Part model, mm, in its own coordinate system. Round coordinates to 2 decimals unless told otherwise and drop trailing zeros. Order: outer loops, then holes, each group sorted by start corner. A loop starts at its lowest first (then second) coordinate and runs counter-clockwise, first axis right, second up. Notation, with made-up numbers: M 71.5,-21 L 101.5,-21 A20 cw 101.5,2 Z; hole C 79,-31 d6. An arc over 180 degrees is marked long. Write each question's results on one line, items separated by ' | '. Start each with the question number.
1. Probe L1, parallel to Z at x = 24, y = 3.75; L2, parallel to X at y = 3, z = 48; L3, parallel to Z at x = 40, y = 6.5. List the from-to ranges inside material, lowest first. Write a range as [from, to].
2. Band-saw the part on D-D, the plane z = -54. List the corners of the cut face in (x, y), then the cut area to 3 significant figures.
3. Band-saw the part on A-A, the plane x = 76. List the corners of the cut face in (y, z).
4. Band-saw the part on B-B, the plane y = 4.5. List the corners of the cut face in (x, z).
5. Band-saw the part on C-C, the plane z = 19. List the corners of the cut face in (x, y).
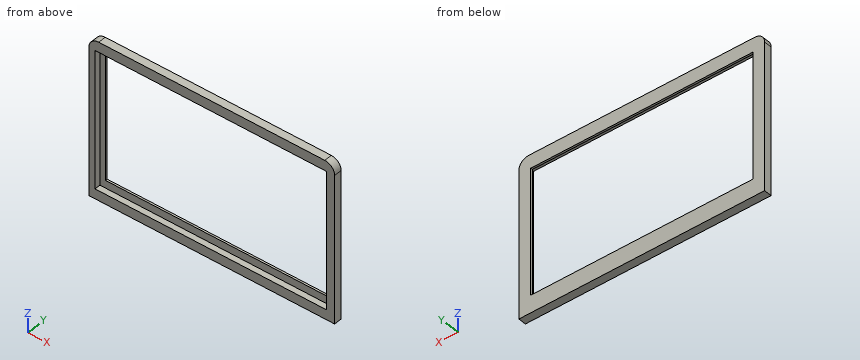
```python
from build123d import *

# Parameters (mm, degrees)
SKETCH_1_W          = 250
SKETCH_1_H          = 156
SKETCH_1_W_2        = 226
SKETCH_1_H_2        = 128
EXTRUDE_1_DEPTH     = 8
SKETCH_2_W          = 235.5
SKETCH_2_H          = 139.5
CUT_EXTRUDE_3_DEPTH = 6
SKETCH_11_W         = 250
SKETCH_11_H         = 8
EXTRUDE_3_DEPTH     = 3.75
CUT_EXTRUDE_4_DEPTH = 10


with BuildPart() as part:
    # 草图1 → 凸台-拉伸1 (new body)
    with BuildSketch(Plane(origin=(0, 0, 0), x_dir=(1, 0, 0), z_dir=(0, 1, 0))):
        with Locations((25.659327926, -14.898030127)):
            Rectangle(SKETCH_1_W, SKETCH_1_H)
        with Locations((25.659327926, -14.898030127)):
            Rectangle(SKETCH_1_W_2, SKETCH_1_H_2, mode=Mode.SUBTRACT)
    extrude(amount=EXTRUDE_1_DEPTH)

    # 草图2 → 切除-拉伸3 (cut)
    with BuildSketch(Plane.XZ):
        with Locations((24.659327926, 12.898030127)):
            Rectangle(SKETCH_2_W, SKETCH_2_H)
    extrude(amount=-CUT_EXTRUDE_3_DEPTH, mode=Mode.SUBTRACT)

    # 草图11 → 凸台-拉伸3 (add)
    with BuildSketch(Plane(origin=(0, 0, -63.101969873), x_dir=(-1, 0, 0), z_dir=(0, 0, -1))):
        with Locations((-25.659327926, 4)):
            Rectangle(SKETCH_11_W, SKETCH_11_H)
    extrude(amount=EXTRUDE_3_DEPTH)

    # 草图12 → 切除-拉伸4 (cut)
    with BuildSketch(Plane(origin=(0, 8, 0), x_dir=(1, 0, 0), z_dir=(0, 1, 0))):
        with BuildLine():
            Line((-99.340672074, -82.898030127), (-99.340672074, -92.898030127))
            Line((-99.340672074, -92.898030127), (-89.340672074, -92.898030127))
            ThreePointArc((-89.340672074, -92.898030127), (-96.411739886, -89.969097939), (-99.340672074, -82.898030127))
        make_face()
        with BuildLine():
            Line((150.659327926, -82.898030127), (150.659327926, -92.898030127))
            Line((150.659327926, -92.898030127), (140.659327926, -92.898030127))
            ThreePointArc((140.659327926, -92.898030127), (147.730395738, -89.969097939), (150.659327926, -82.898030127))
        make_face()
    extrude(amount=-CUT_EXTRUDE_4_DEPTH, mode=Mode.SUBTRACT)


solid = part.part
```
Solution:
1) L1: [-66.85, -56.85], [82.65, 92.9] | L2: [-99.34, -93.09], [142.41, 150.66] | L3: [-66.85, -49.1], [78.9, 92.9]
2) outline: M -99.34,0 L -93.09,0 L -93.09,6 L 142.41,6 L 142.41,0 L 150.66,0 L 150.66,8 L -99.34,8 Z | area: 587 mm^2
3) outline: M 0,-66.85 L 8,-66.85 L 8,-49.1 L 6,-49.1 L 6,-56.85 L 0,-56.85 Z; M 0,82.65 L 6,82.65 L 6,78.9 L 8,78.9 L 8,92.9 L 0,92.9 Z
4) outline: M -99.34,-66.85 L 150.66,-66.85 L 150.66,82.9 A10 ccw 140.66,92.9 L -89.34,92.9 A10 ccw -99.34,82.9 Z; hole M -93.09,-56.85 L 142.41,-56.85 L 142.41,82.65 L -93.09,82.65 Z
5) outline: M -99.34,0 L -93.09,0 L -93.09,6 L -87.34,6 L -87.34,8 L -99.34,8 Z; M 138.66,6 L 142.41,6 L 142.41,0 L 150.66,0 L 150.66,8 L 138.66,8 Z
